```python
from build123d import *

# Parameters (mm, degrees)
SKETCH018_W             = 126
SKETCH018_H             = 68
PAD008_DEPTH            = 3
SKETCH019_W             = 6
SKETCH019_H             = 12
PAD009_DEPTH            = 13.5
SKETCH020_R             = 2.25
POCKET009_DEPTH         = 122.851
POCKET010_DEPTH         = 3.5
SKETCH022_W             = 10.5
SKETCH022_H             = 12.5
POCKET011_DEPTH         = 16.501
CHAMFER002_SIZE         = 1
CHAMFER007_SIZE         = 1
CHAMFER009_SIZE         = 1
PAD015_DEPTH            = 2
BODY005_PLACEMENT_ANGLE = 180


with BuildPart() as part:
    # Sketch018 → Pad008 (new body)
    with BuildSketch(Plane.XZ):
        with Locations((0, 34)):
            Rectangle(SKETCH018_W, SKETCH018_H)
    extrude(amount=PAD008_DEPTH)

    # Sketch019 (on Face5 of Pad008) → Pad009 (join)
    with BuildSketch(Plane(origin=(0, 0, 0), x_dir=(1, 0, 0), z_dir=(0, 1, 0))):
        with Locations((-56.85, -16)):
            Rectangle(SKETCH019_W, SKETCH019_H)
        with Locations((-56.85, -52)):
            Rectangle(SKETCH019_W, SKETCH019_H)
    pad009 = extrude(amount=PAD009_DEPTH)

    # Mirrored004: Pad009 across YZ
    add(pad009.mirror(Plane.YZ))

    # Sketch020 (on Face22 of Mirrored004) → Pocket009 (cut, through all)
    with BuildSketch(Plane(origin=(59.85, 0, 0), x_dir=(0, 0, 1), z_dir=(1, 0, 0))):
        with Locations((16, -7)):
            Circle(SKETCH020_R)
        with Locations((52, -7)):
            Circle(SKETCH020_R)
    extrude(amount=-POCKET009_DEPTH, mode=Mode.SUBTRACT)

    # Sketch021 (on Face10 of Pocket009) → Pocket010 (cut)
    with BuildSketch(Plane(origin=(-53.85, 0, 0), x_dir=(0, 0, 1), z_dir=(1, 0, 0))):
        Polygon((19.5, -9.020726), (19.5, -4.979274), (16, -2.958548), (12.5, -4.979274), (12.5, -9.020726), (16, -11.041452), align=None)
        Polygon((55.5, -9.020726), (55.5, -4.979274), (52, -2.958548), (48.5, -4.979274), (48.5, -9.020726), (52, -11.041452), align=None)
    pocket010 = extrude(amount=-POCKET010_DEPTH, mode=Mode.SUBTRACT)

    # Sketch022 (on Face5 of Pocket010) → Pocket011 (cut, through all)
    with BuildSketch(Plane.XZ.offset(3)):
        with Locations((16, 18.25)):
            Rectangle(SKETCH022_W, SKETCH022_H)
    extrude(amount=-POCKET011_DEPTH, mode=Mode.SUBTRACT)

    # Chamfer002
    chamfer002_edges = [part.edges().sort_by_distance(p)[0] for p in [
        (0, -3, 68),
        (-63, -3, 34),
        (63, -3, 34),
        (0, -3, 0),
        (16, -3, 24.5),
        (21.25, -3, 18.25),
        (16, -3, 12),
        (10.75, -3, 18.25),
    ]]
    chamfer(chamfer002_edges, length=CHAMFER002_SIZE)

    # Chamfer007
    chamfer007_edges = [part.edges().sort_by_distance(p)[0] for p in [
        (-63, -1, 68),
        (63, -1, 68),
    ]]
    chamfer(chamfer007_edges, length=CHAMFER007_SIZE)

    # Chamfer009
    chamfer009_edges = [part.edges().sort_by_distance(p)[0] for p in [
        (-63, -1, 0),
        (63, -1, 0),
    ]]
    chamfer(chamfer009_edges, length=CHAMFER009_SIZE)

    # Mirrored006: Pocket010 across YZ
    add(pocket010.mirror(Plane.YZ), mode=Mode.SUBTRACT)

    # Sketch034 (on Face1 of Mirrored006) → Pad015 (join)
    with BuildSketch(Plane(origin=(0, 0, 0), x_dir=(1, 0, 0), z_dir=(0, 1, 0))):
        with BuildLine():
            ThreePointArc((-22.5, -4.5), (-24, -6), (-22.5, -7.5))
            Line((-22.5, -7.5), (22.5, -7.5))
            ThreePointArc((22.5, -7.5), (24, -6), (22.5, -4.5))
            Line((-22.5, -4.5), (22.5, -4.5))
        make_face()
        with BuildLine():
            ThreePointArc((-47.5, -33.5), (-49, -35), (-47.5, -36.5))
            Line((-47.5, -36.5), (47.5, -36.5))
            ThreePointArc((47.5, -36.5), (49, -35), (47.5, -33.5))
            Line((-47.5, -33.5), (47.5, -33.5))
        make_face()
    extrude(amount=PAD015_DEPTH)


with BuildPart() as part_1:
    # Body005 placement: moved
    add(part.part.moved(Location((0, 66.95, 0))).rotate(Axis((0, 66.95, 0), (0, 0, 1)), BODY005_PLACEMENT_ANGLE))


solid = part_1.part
```
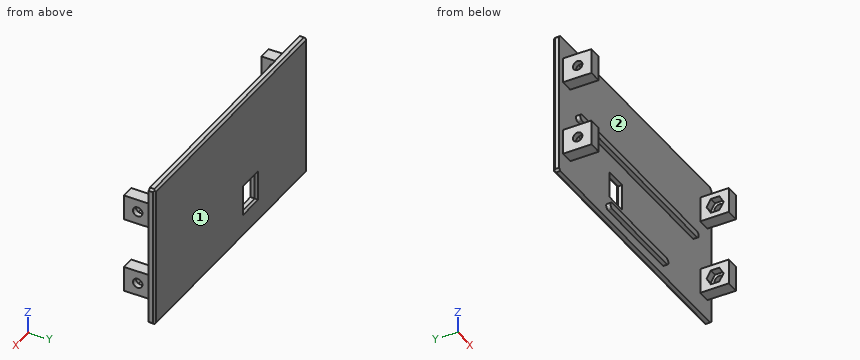
Work out the finished part from the listing and answer in its coordinate system (mm). Face numbers are marked on the shaded views. Coordinates: 2 decimals unless noted, no trailing zeros. Loops run counter-clockwise (first coordinate to the right, second up) from the corner with the lowest first, then second, coordinate; pieces in that order, holes last. Notation, with made-up numbers: (26.5, 71.25) - (57.5, 71.25) arc R36 cw to (57.5, 109.25) - close; hole circle Ø3 at (-34.75, 16.25). An arc over 180 degrees is marked (long way). Use a Markdown table: item, result.
Item 1: Find section C-C, the plane z = 30. Determine the outline of the cut face in (x, y), and give its area (3 significant figures).
Evaluation:
| item | result |
|---|---|
| outline | (-63, 66.95) - (63, 66.95) - (63, 68.95) - (62, 69.95) - (-62, 69.95) - (-63, 68.95) - close |
| area | 377 mm2 |
Item 2: Find section A-A, the plane x = -6. Determine the outline of the cut face in (y, z), and give its area (3 significant figures).
Evaluation:
| item | result |
|---|---|
| outline | (64.95, 4.5) - (66.95, 4.5) - (66.95, 0) - (68.95, 0) - (69.95, 1) - (69.95, 67) - (68.95, 68) - (66.95, 68) - (66.95, 36.5) - (64.95, 36.5) - (64.95, 33.5) - (66.95, 33.5) - (66.95, 7.5) - (64.95, 7.5) - close |
| area | 215 mm2 |
Item 3: Consider probe 1 along Z at (x, y) = (59.2, 59.95); probe 2 along Z at (x, y) = (-56, 59.5); probe 3 along Y at (x, z) = (-59, 16). Determine where each line is inside the solid, lowest interval first. Write a range as from..to.
Evaluation:
| item | result |
|---|---|
| probe 1 | z = 10..13.75, 18.25..22, 46..49.75, 54.25..58 |
| probe 2 | z = 10..12.5, 19.5..22, 46..48.5, 55.5..58 |
| probe 3 | y = 53.45..57.7, 62.2..69.95 |
Item 4: Find section D-D, the plane x = 34. Determine the outline of the cut face in (y, z).
Evaluation:
| item | result |
|---|---|
| outline | (64.95, 33.5) - (66.95, 33.5) - (66.95, 0) - (68.95, 0) - (69.95, 1) - (69.95, 67) - (68.95, 68) - (66.95, 68) - (66.95, 36.5) - (64.95, 36.5) - close |
Item 5: Given pin 1 Ø3 at (x, z) = (-35, 9.5) entering from -Y; pin 2 Ø9.5 at (y, z) = (62, 16.5) entering from -X; pin 3 Ø1 at (x, y) = (-56, 59) entering from +Z, each flat-ended and moving along its own axis, determine where each tip first touches the part or whether it passes through.
Evaluation:
| item | result |
|---|---|
| pin 1 | stops at y = 66.95 |
| pin 2 | stops at x = -59.85 |
| pin 3 | stops at z = 58 |
Item 6: Find section B-B, the plane z = 6. Determine the outline of the cut face in (x, y), and give its area (3 significant figures).
Evaluation:
| item | result |
|---|---|
| outline | (-63, 66.95) - (-24, 66.95) - (-24, 64.95) - (24, 64.95) - (24, 66.95) - (63, 66.95) - (63, 68.95) - (62, 69.95) - (-62, 69.95) - (-63, 68.95) - close |
| area | 473 mm2 |
Item 7: The mould has two halves that part along X. Classify the marked faces 1 and 2: +X half, -X half, draft (parallel to the pull), parting line (faces both ways), or undercut.
Evaluation:
| item | result |
|---|---|
| face 1 | draft |
| face 2 | undercut |
